from build123d import *

# Parameters (mm, degrees)
SKETCH1_R           = 8
BOSS_EXTRUDE1_DEPTH = 2.2
SKETCH2_R           = 1.3
CUT_EXTRUDE1_DEPTH  = 2.2
SKETCH3_R           = 3
SKETCH3_R_2         = 2.45
BOSS_EXTRUDE2_DEPTH = 2.2
SKETCH8_R           = 0.6
CUT_EXTRUDE7_DEPTH  = 2.2
CUT_EXTRUDE8_START  = -1.7
SKETCH9_R           = 2.45
CUT_EXTRUDE8_DEPTH  = 1.7


with BuildPart() as part:
    # Sketch1 → Boss-Extrude1 (new body)
    with BuildSketch(Plane(origin=(0, 0, 0), x_dir=(1, 0, 0), z_dir=(0, 1, 0))):
        with Locations(Location((0, 0, 0), (0, 0, 270))):
            Circle(SKETCH1_R)
    extrude(amount=BOSS_EXTRUDE1_DEPTH)

    # Sketch2 → Cut-Extrude1 (cut)
    with BuildSketch(Plane(origin=(0, 2.2, 0), x_dir=(1, 0, 0), z_dir=(0, 1, 0))):
        with Locations(Location((0, 4.5, 0), (0, 0, 270))):
            Circle(SKETCH2_R)
        with Locations(Location((0, -4.5, 0), (0, 0, 90))):
            Circle(SKETCH2_R)
    extrude(amount=-CUT_EXTRUDE1_DEPTH, mode=Mode.SUBTRACT)

    # Sketch3 → Boss-Extrude2 (add)
    with BuildSketch(Plane.XZ):
        with Locations(Location((0, 0, 0), (0, 0, 90))):
            Circle(SKETCH3_R)
        with Locations(Location((0, 0, 0), (0, 0, 270))):
            Circle(SKETCH3_R_2, mode=Mode.SUBTRACT)
    extrude(amount=BOSS_EXTRUDE2_DEPTH)

    # Sketch8 → Cut-Extrude7 (cut)
    with BuildSketch(Plane.XZ):
        with Locations(Location((0, 0, 0), (0, 0, 270))):
            Circle(SKETCH8_R)
    extrude(amount=-CUT_EXTRUDE7_DEPTH, mode=Mode.SUBTRACT)

    # Sketch9 → Cut-Extrude8 (cut)
    with BuildSketch(Plane.XZ.offset(CUT_EXTRUDE8_START)):
        with Locations(Location((0, 0, 0), (0, 0, 270))):
            Circle(SKETCH9_R)
    extrude(amount=CUT_EXTRUDE8_DEPTH, mode=Mode.SUBTRACT)


solid = part.part
The model under review builds one solid part; all positions refer to its coordinate system, in mm. A direction names the side the tool comes from. Give positions to 0.01 mm unless a question says otherwise; leave off trailing zeros. Loops run counter-clockwise (first coordinate to the right, second up) from the corner with the lowest first, then second, coordinate; pieces in that order, holes last. Notation, with made-up numbers: (80.5, 64.25) -> (106.5, 64.25) arc R19 cw to (106.5, 79.25) -> close; hole circle Ø10 at (18.25, 44). An arc over 180 degrees is marked (long way). Answer as a JSON object with one key per item and string values. Group by question number.
Q1. Insertion check: pin 1 (1 mm diameter, centred on x = 0, z = 0, fed in from +Y); pin 2 (1 mm diameter, centred on x = -2.5, y = 0.5, fed in from -Z); pin 3 (2.5 mm diameter, centred on x = -0.5, z = 0, fed in from -Y). Each pin has a flat end and moves straight along its axis. Give the tip position at first contact, or say it passes through.
Q2. Wall thickness on line 1 along Z through (x, y) = (0.25, 0.2); line 2 along X through (y, z) = (2.1, 0); line 3 along X through (y, z) = (1.25, 0): over which ranges is each line inside the solid? List them lowest first.
Q3. Take a section at B-B (z = 0). Write out the cut boundary in (x, y).
Q4. Draft analysis for pull direction Z (two halves, no side actions). For faces 3 (the cylindrical face through (-7.81, 1.08, -1.73)), 4 (the flat face through (-3.4, 0, -0.1)), 5 (the cylindrical face through (0.506, 1.947, -0.323)), state which applies: pulls with the +Z half, pulls with the -Z half, needs draft (parallel to the pull), parting line crosses it, or undercut.
Q5. Take a section at D-D (y = 0.25). Write out the cut boundary in (x, z), plus the area to 3 significant figures.
Q6. Take a section at A-A (x = 0). Write out the cut boundary in (y, z), plus the area to 4 significant figures.
Q7. Take a section at C-C (z = 5.25). Write out the cut boundary in (x, y), plus the area to 3 significant figures.
Q8. Tool access review of faces 1 (the cylindrical face through (-0.39, 1.12, 3.26)), 2 (the flat face through (-1, 1.7, -1)): name each direction out of +Z, -Z, +X, -X, +Y, -Y from which nothing blocks a thin tool from reaching the whole face with its end or side.
Answer below:
{
 "1": {"pin 1": "passes through", "pin 2": "stops at z = -7.75", "pin 3": "stops at y = 1.7"},
 "2": {"line 1": "z = -8 to -5.78, -3.22 to -2.44, 2.44 to 3.22, 5.78 to 8", "line 2": "x = -8 to -0.6, 0.6 to 8", "line 3": "x = -8 to -2.45, 2.45 to 8"},
 "3": {"outline": "(-8, 0) -> (-3, 0) -> (-3, -2.2) -> (-2.45, -2.2) -> (-2.45, 1.7) -> (-0.6, 1.7) -> (-0.6, 2.2) -> (-8, 2.2) -> close; (0.6, 1.7) -> (2.45, 1.7) -> (2.45, -2.2) -> (3, -2.2) -> (3, 0) -> (8, 0) -> (8, 2.2) -> (0.6, 2.2) -> close"},
 "4": {"face 3": "parting line crosses it", "face 4": "needs draft", "face 5": "undercut"},
 "5": {"outline": "circle Ø16 at (0, 0); hole circle Ø4.9 at (0, 0); hole circle Ø2.6 at (0, -4.5); hole circle Ø2.6 at (0, 4.5)", "area": "172 mm2"},
 "6": {"outline": "(-2.2, -3) -> (0, -3) -> (0, -3.2) -> (2.2, -3.2) -> (2.2, -0.6) -> (1.7, -0.6) -> (1.7, -2.45) -> (-2.2, -2.45) -> close; (-2.2, 2.45) -> (1.7, 2.45) -> (1.7, 0.6) -> (2.2, 0.6) -> (2.2, 3.2) -> (0, 3.2) -> (0, 3) -> (-2.2, 3) -> close; (0, -8) -> (2.2, -8) -> (2.2, -5.8) -> (0, -5.8) -> close; (0, 5.8) -> (2.2, 5.8) -> (2.2, 8) -> (0, 8) -> close", "area": "17.25 mm2"},
 "7": {"outline": "(-6.04, 0) -> (-1.06, 0) -> (-1.06, 2.2) -> (-6.04, 2.2) -> close; (1.06, 0) -> (6.04, 0) -> (6.04, 2.2) -> (1.06, 2.2) -> close", "area": "21.9 mm2"},
 "8": {"face 1": "+Y, -Y", "face 2": "-Y"}
}
